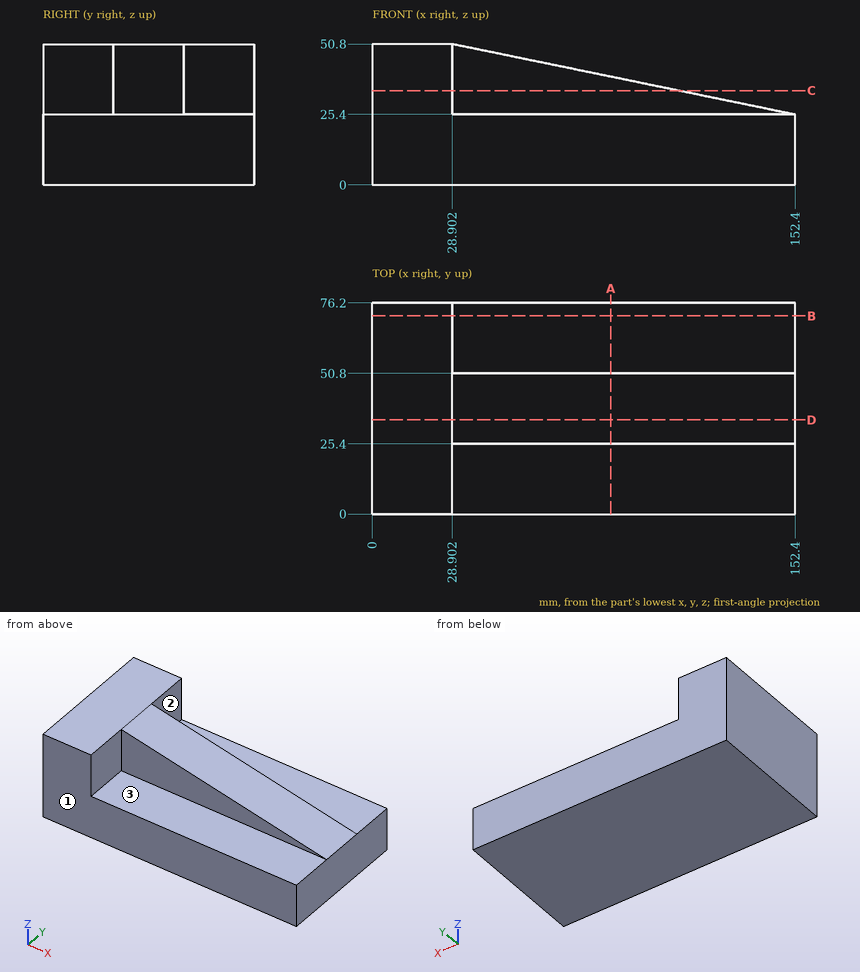
Verification items for this drawing (mm, ordinates from the low corner). A direction names the side the tool comes from. Coordinates: 2 decimals unless noted, no trailing zeros. Loops run counter-clockwise (first coordinate to the right, second up) from the corner with the lowest first, then second, coordinate; pieces in that order, holes last. Notation, with made-up numbers: (65, 7.25) - (70, 7.25) arc R24 cw to (70, 27.25) - close; hole circle Ø6 at (25, 64). An arc over 180 degrees is marked (long way). Use one line per item in the form item = value. Start each with the question number.
Item 1: Section check D-D, the plane y = 34. Enter the section's corners in (x, z).
Item 2: Gauge pin test, flat ends, axial feed: pin 1 (5 mm diameter, centred on x = 31.5, y = 62, fed in from +Z); pin 2 (3 mm diameter, centred on x = 41.5, y = 21, fed in from -Z); pin 3 (8 mm diameter, centred on x = 89, y = 47.5, fed in from +Z); pin 4 (12.5 mm diameter, centred on x = 92, z = 42.5, fed in from +Y). Record the tip position at first contact, or that the pin passes through.
Item 3: Section check C-C, the plane z = 34. Enter the section's corners in (x, y) (1 decimal).
Item 4: Tool access check on the marked faces 1, 2 and 3. Record the directions out of +Z, -Z, +X, -X, +Y, -Y that give a thin tool (end or side, any length) a straight path to the whole face; none if there is none.
Item 5: Thickness scan on probe 1 along Z at (x, y) = (127.5, 22); probe 2 along Y at (x, z) = (55, 38); probe 3 along X at (y, z) = (4.5, 31.5). Record the ranges inside material, lowest first.
Item 6: Section check A-A, the plane x = 86. Enter the section's corners in (y, z), and give its area (3 significant figures).
Item 7: Section check B-B, the plane y = 71.5. Enter the section's corners in (x, z).
Computed:
q1.outline = (0, 0) - (152.4, 0) - (152.4, 25.4) - (28.9, 50.8) - (0, 50.8) - close
q2.pin_1 = 25.4
q2.pin_2 = 0
q2.pin_3 = 39.26
q2.pin_4 = 50.8
q3.outline = (0, 0) - (28.9, 0) - (28.9, 25.4) - (110.6, 25.4) - (110.6, 50.8) - (28.9, 50.8) - (28.9, 76.2) - (0, 76.2) - close
q4.face_1 = +Z, -Z, +X, -X, -Y
q4.face_2 = +Z, +X, +Y
q4.face_3 = +Z, +X, -Y
q5.probe_1 = 0 to 25.4
q5.probe_2 = 25.4 to 50.8
q5.probe_3 = 0 to 28.9
q6.outline = (0, 0) - (76.2, 0) - (76.2, 25.4) - (50.8, 25.4) - (50.8, 39.06) - (25.4, 39.06) - (25.4, 25.4) - (0, 25.4) - close
q6.area = 2,280 mm2
q7.outline = (0, 0) - (152.4, 0) - (152.4, 25.4) - (28.9, 25.4) - (28.9, 50.8) - (0, 50.8) - close
